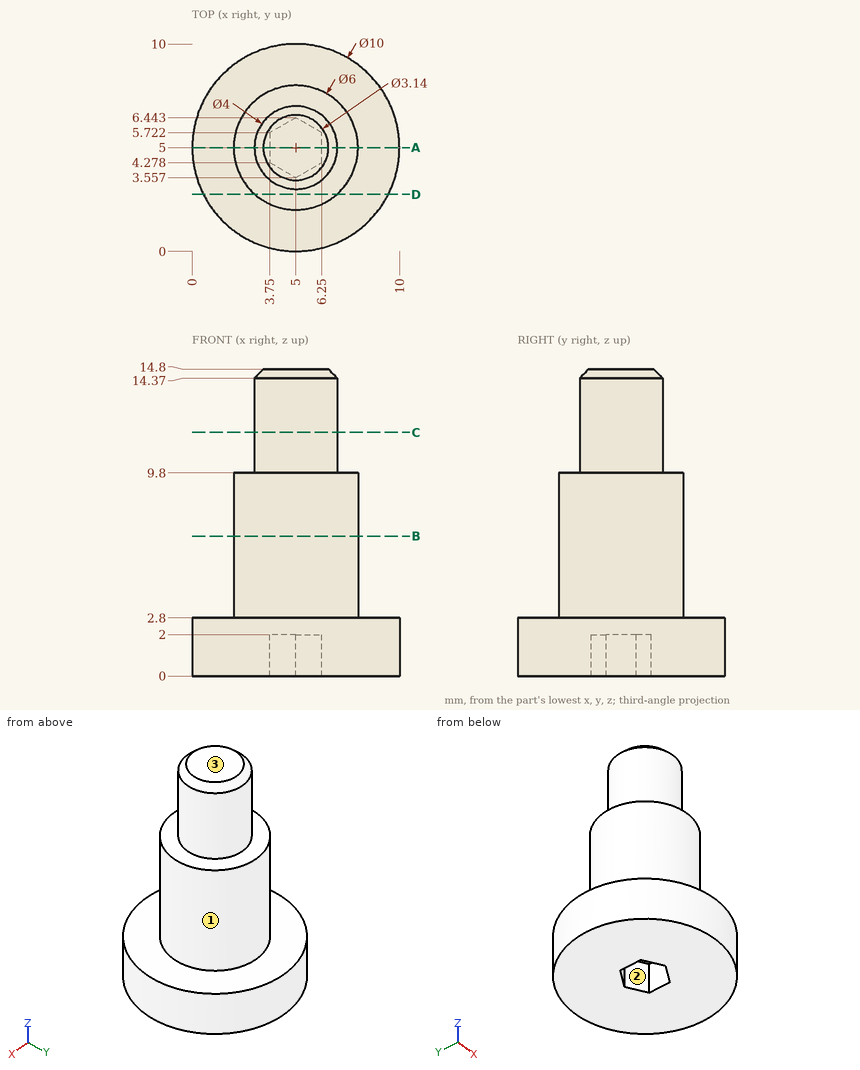
The figure shows three views and two pictorial views of one solid part (mm, origin at its lowest corner). Answer the questions. A direction names the side the tool comes from. Give positions to 0.01 mm unless a question says otherwise; leave off trailing zeros. Write each loop counter-clockwise with the first axis right and the second up, starting at its lowest first coordinate (ties: lowest second). Pieces come first, ordered by that corner, then holes.
Q1. The part is cut by section B-B on z = 6.75. Give the vertices of the cut face in (x, y).
Answer:
outline: circle Ø6 at (5, 5)
Q2. The part is cut by section C-C on z = 11.75. Give the vertices of the cut face in (x, y), and give its area (3 significant figures).
Answer:
outline: circle Ø4 at (5, 5)
area: 12.6 mm2
Q3. Straight lines are drawn through the part: L1, parallel to Z at x = 5, y = 8.25; L2, parallel to Z at x = 2.25, y = 4.25; L3, parallel to Y at x = 5.75, z = 1.75 (1 decimal). For each, find the intervals that lie inside material, in ascending order.
Answer:
L1: z = 0 to 2.8
L2: z = 0 to 9.8
L3: y = 0.1 to 4, 6 to 9.9
Q4. The part is cut by section D-D on y = 2.75. Give the vertices of the cut face in (x, z) (1 decimal).
Answer:
outline: (0.5, 0) - (9.5, 0) - (9.5, 2.8) - (7, 2.8) - (7, 9.8) - (3, 9.8) - (3, 2.8) - (0.5, 2.8) - close
Q5. Given pin 1 (1.5 mm diameter, centred on x = 2.5, y = 3.5, fed in from +Z); pin 2 (5 mm diameter, centred on y = 2, z = 7.5, fed in from -X); pin 3 (5 mm diameter, centred on x = 7, y = 4, fed in from -Z); pin 4 (1.3 mm diameter, centred on x = 5, y = 5.5, fed in from -Z), each flat-ended and moving along its own axis, determine where each tip first touches the part or whether it passes through.
Answer:
pin 1: stops at z = 9.8
pin 2: stops at x = 2.04
pin 3: stops at z = 0
pin 4: stops at z = 2
Q6. The part is cut by section A-A on y = 5. Give the vertices of the cut face in (x, z).
Answer:
outline: (0, 0) - (3.75, 0) - (3.75, 2) - (6.25, 2) - (6.25, 0) - (10, 0) - (10, 2.8) - (8, 2.8) - (8, 9.8) - (7, 9.8) - (7, 14.37) - (6.57, 14.8) - (3.43, 14.8) - (3, 14.37) - (3, 9.8) - (2, 9.8) - (2, 2.8) - (0, 2.8) - close
Q7. A tool of negligible diameter and unlimited length cuts with its end or side. For the marked faces 1, 2 and 3, from which of +Z, -Z, +X, -X, +Y, -Y can it reach the whole face along a straight path? Write none if from no direction.
Answer:
face 1: +Z
face 2: -Z
face 3: +Z, +X, -X, +Y, -Y
